The listing builds one solid part. Answer for the finished solid, in the listing's coordinates (mm). A direction names the side the tool comes from. Coordinates: 2 decimals unless noted, no trailing zeros. Write each loop counter-clockwise with the first axis right and the second up, starting at its lowest first coordinate (ties: lowest second). Pieces come first, ordered by that corner, then holes.
from build123d import *

# Parameters (mm, degrees)
SKETCH2_R           = 1.25
SKETCH2_R_2         = 5.1
BOSS_EXTRUDE2_DEPTH = 4.5
FILLET1_R           = 10
SKETCH4_R           = 2
CUT_EXTRUDE1_DEPTH  = 2
SKETCH5_R           = 12.5
SKETCH5_R_2         = 1.25
BOSS_EXTRUDE3_DEPTH = 2.5
SKETCH8_R           = 5.1
CUT_EXTRUDE5_DEPTH  = 10


with BuildPart() as part:
    # Sketch2 → Boss-Extrude2 (new body)
    with BuildSketch(Plane(origin=(0, 0, 0), x_dir=(1, 0, 0), z_dir=(0, 1, 0))):
        with BuildLine():
            Line((6.75, -45), (6.75, -10.520812706))
            ThreePointArc((6.75, -10.520812706), (0, 12.5), (-6.75, -10.520812706))
            Line((-6.75, -10.520812706), (-6.75, -45))
            ThreePointArc((-6.75, -45), (0, -51.75), (6.75, -45))
        make_face()
        with Locations((8, 0)):
            Circle(SKETCH2_R, mode=Mode.SUBTRACT)
        with Locations((0, -8)):
            Circle(SKETCH2_R, mode=Mode.SUBTRACT)
        with Locations((-8, 0)):
            Circle(SKETCH2_R, mode=Mode.SUBTRACT)
        with Locations((0, 8)):
            Circle(SKETCH2_R, mode=Mode.SUBTRACT)
        with Locations((0, -45)):
            Circle(SKETCH2_R_2, mode=Mode.SUBTRACT)
    extrude(amount=BOSS_EXTRUDE2_DEPTH)

    # Fillet1
    fillet1_edges = [part.edges().sort_by_distance(p)[0] for p in [
        (-6.75, 2.25, 10.520812706),
        (6.75, 2.25, 10.520812706),
    ]]
    fillet(fillet1_edges, radius=FILLET1_R)

    # Sketch4 → Cut-Extrude1 (cut)
    with BuildSketch(Plane.XZ):
        with Locations((0, 8)):
            Circle(SKETCH4_R)
        with Locations((-8, 0)):
            Circle(SKETCH4_R)
        with Locations((8, 0)):
            Circle(SKETCH4_R)
        with Locations((0, -8)):
            Circle(SKETCH4_R)
    extrude(amount=-CUT_EXTRUDE1_DEPTH, mode=Mode.SUBTRACT)

    # Sketch5 → Boss-Extrude3 (add)
    with BuildSketch(Plane(origin=(0, 4.5, 0), x_dir=(1, 0, 0), z_dir=(0, 1, 0))):
        Circle(SKETCH5_R)
        with Locations((8, 0)):
            Circle(SKETCH5_R_2, mode=Mode.SUBTRACT)
        with Locations((0, 8)):
            Circle(SKETCH5_R_2, mode=Mode.SUBTRACT)
        with Locations((-8, 0)):
            Circle(SKETCH5_R_2, mode=Mode.SUBTRACT)
        with Locations((0, -8)):
            Circle(SKETCH5_R_2, mode=Mode.SUBTRACT)
    extrude(amount=BOSS_EXTRUDE3_DEPTH)

    # Sketch8 → Cut-Extrude5 (cut)
    with BuildSketch(Plane.XZ):
        Circle(SKETCH8_R)
    extrude(amount=-CUT_EXTRUDE5_DEPTH, mode=Mode.SUBTRACT)


solid = part.part
Q1. Find the intervals of material crossed by probe 1 along Z at (x, y) = (0, 0.9); probe 2 along Z at (x, y) = (0, 5.05); probe 3 along Z at (x, y) = (0, 4.25), in increasing order.
Answers below:
probe 1: z = -12.5 to -10, -6 to -5.1, 5.1 to 6, 10 to 39.9, 50.1 to 51.75
probe 2: z = -12.5 to -9.25, -6.75 to -5.1, 5.1 to 6.75, 9.25 to 12.5
probe 3: z = -12.5 to -9.25, -6.75 to -5.1, 5.1 to 6.75, 9.25 to 39.9, 50.1 to 51.75
Q2. Given pin 1 (3 mm diameter, centred on y = 3, z = 36, fed in from +X); pin 2 (2 mm diameter, centred on y = 2.5, z = 30, fed in from -X); pin 3 (6 mm diameter, centred on x = -6.5, z = 33.5, fed in from +Y), each flat-ended and moving along its own axis, determine where each tip first touches the part or whether it passes through.
Answers below:
pin 1: stops at x = 6.75
pin 2: stops at x = -6.75
pin 3: stops at y = 4.5
Q3. The part is cut by section C-C, the plane y = 0.75. Write down the section's boundary in (x, z), then the cut area to 3 significant figures.
Answers below:
outline: (-9.31, 8.35) arc R12.5 ccw (long way) to (9.31, 8.35) arc R10 cw to (6.75, 15.02) - (6.75, 45) arc R6.75 ccw to (-6.75, 45) - (-6.75, 15.02) arc R10 cw to start; hole circle Ø4 at (-8, 0); hole circle Ø10.2 at (0, 0); hole circle Ø10.2 at (0, 45); hole circle Ø4 at (0, -8); hole circle Ø4 at (0, 8); hole circle Ø4 at (8, 0)
area: 801 mm2
Q4. The part is cut by section D-D, the plane z = -8. Write down the section's boundary in (x, y), then the cut area to 3 significant figures.
Answers below:
outline: (-9.6, 0) - (-2, 0) - (-2, 2) - (-1.25, 2) - (-1.25, 7) - (-9.6, 7) - close; (1.25, 2) - (2, 2) - (2, 0) - (9.6, 0) - (9.6, 7) - (1.25, 7) - close
area: 114 mm2
Q5. The part is cut by section B-B, the plane z = 0. Write down the section's boundary in (x, y), then the cut area to 3 significant figures.
Answers below:
outline: (-12.5, 0) - (-10, 0) - (-10, 2) - (-9.25, 2) - (-9.25, 7) - (-12.5, 7) - close; (-6.75, 2) - (-6, 2) - (-6, 0) - (-5.1, 0) - (-5.1, 7) - (-6.75, 7) - close; (5.1, 0) - (6, 0) - (6, 2) - (6.75, 2) - (6.75, 7) - (5.1, 7) - close; (9.25, 2) - (10, 2) - (10, 0) - (12.5, 0) - (12.5, 7) - (9.25, 7) - close
area: 62.6 mm2
Q6. Which of the six approach directions +Z, -Z, +X, -X, +Y, -Y give full straight-line access (tool end or side, diameter ignored) to faces 4 (the face through (1, 2, -7)), 5 (the face through (-6.75, 2, 30)), 6 (the face through (0, 0, 12))?
Answers below:
face 4: -Y
face 5: +Z, -X, +Y, -Y
face 6: +Z, -Z, +X, -X, -Y
Q7. The part is cut by section A-A, the plane x = 0. State how many separate pieces and enclosed holes the cut face has, then the cut area to 3 significant figures.
Answers below:
separate pieces: 5
enclosed holes: 0
area: 193 mm2
Q8. Determine the mould class of faces 1 (the face through (-0.2, 7, 5.4)), 2 (the face through (6.75, 2, 30)), 3 (the face through (2.4, 2.2, 49.5)) for opening direction X: released by +X, released by -X, zero draft, split by the parting line, or undercut.
Answers below:
face 1: zero draft
face 2: released by +X
face 3: undercut
